from build123d import *

# Parameters (mm, degrees)
SKETCH1_R               = 10
BOSS_EXTRUDE1_DEPTH     = 15
SKETCH2_R               = 12.5
BOSS_EXTRUDE2_DEPTH     = 20
SKETCH3_R               = 12
BOSS_EXTRUDE3_DEPTH     = 139.5
SKETCH4_R               = 4.5
CUT_EXTRUDE1_DEPTH      = 176.393129854
CUT_EXTRUDE2_DEPTH      = 176.393129954
CUT_EXTRUDE2_DEPTH_BACK = 176.393129954
SKETCH5_W               = 50.129657838
SKETCH5_H               = 19.874218845
LPATTERN1_COUNT         = 2
LPATTERN1_PITCH         = 25


with BuildPart() as part:
    # Sketch1 → Boss-Extrude1 (new body)
    with BuildSketch(Plane.XY):
        Circle(SKETCH1_R)
    extrude(amount=BOSS_EXTRUDE1_DEPTH)

    # Sketch2 → Boss-Extrude2 (add)
    with BuildSketch(Plane.XY.offset(15)):
        Circle(SKETCH2_R)
    extrude(amount=BOSS_EXTRUDE2_DEPTH)

    # Sketch3 → Boss-Extrude3 (add)
    with BuildSketch(Plane.XY.offset(35)):
        Circle(SKETCH3_R)
    extrude(amount=BOSS_EXTRUDE3_DEPTH)

    # Sketch4 → Cut-Extrude1 (cut, symmetric)
    with BuildSketch(Plane(origin=(0, 0, 0), x_dir=(1, 0, 0), z_dir=(0, 1, 0))):
        with Locations(Location((0, -154.5, 0), (0, 0, 270))):
            Circle(SKETCH4_R)
    cut_extrude1 = extrude(amount=CUT_EXTRUDE1_DEPTH, both=True, mode=Mode.SUBTRACT)

    # Sketch5 → Cut-Extrude2 (cut, two sides: drawn at the far end of the back side and taken through both)
    with BuildSketch(Plane(origin=(0, 0, 0), x_dir=(1, 0, 0), z_dir=(0, 1, 0)).offset(-CUT_EXTRUDE2_DEPTH_BACK)):
        with Locations((-12.564828919, -5.062890578)):
            Rectangle(SKETCH5_W, SKETCH5_H)
    extrude(amount=CUT_EXTRUDE2_DEPTH + CUT_EXTRUDE2_DEPTH_BACK, mode=Mode.SUBTRACT)

    # LPattern1: Cut-Extrude1 ×2
    with Locations(*[(0, 0, -i * LPATTERN1_PITCH) for i in range(1, LPATTERN1_COUNT)]):
        add(cut_extrude1, mode=Mode.SUBTRACT)


solid = part.part
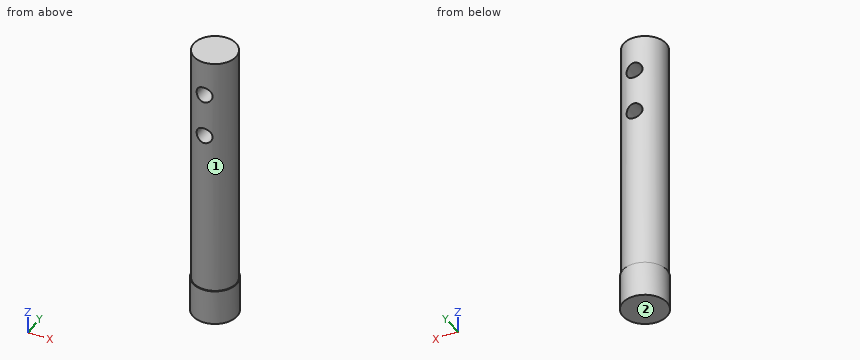
Geometry: final body of the model. Coordinates: model frame, mm. Face numbers are marked on the shaded views. A direction names the side the tool comes from. Coordinates: 2 decimals unless noted, no trailing zeros. Loops run counter-clockwise (first coordinate to the right, second up) from the corner with the lowest first, then second, coordinate; pieces in that order, holes last. Notation, with made-up numbers: (88, 79) - (144, 79) arc R6 ccw to (144, 88) - close; hole circle Ø5 at (-24.75, 2.25). An arc over 180 degrees is marked (long way). Put each result on its own line as item: value. Start each with the question number.
Q1. Line query: line 1 (Z direction, x = 0.5, y = -1.25); line 2 (Z direction, x = -2, y = 5.25); line 3 (X direction, y = -0.5, z = 154.5). Output: solid intervals per line, ascending.
Q2. Set-up query: the marked faces 1 and 2. Return all of +Z, -Z, +X, -X, +Y, -Y with unobstructed straight access to the full face (end or side cutting, diameter ignored); none if empty.
Q3. Pin query (flat end, axial travel): pin 1 Ø14.5 at (x, z) = (0, 129.5) entering from -Y; pin 2 Ø6 at (y, z) = (9, 122) entering from +X; pin 3 Ø5 at (y, z) = (2.5, 105.5) entering from +X. Return the tip coordinate at first contact, or that it passes through.
Q4. Cut plane D-D, the plane y = 6.5. Return loops of the section in (x, z), and give its area (3 significant figures).
Q5. Cut plane C-C, the plane z = 129.5. Return loops of the section in (x, y).
Q6. Cut plane B-B, the plane y = 0. Return loops of the section in (x, z).
Q7. Cut plane A-A, the plane x = 0. Return loops of the section in (y, z).
Filled sheet:
1. line 1: 15 to 125.03, 133.97 to 150.03, 158.97 to 174.5
1. line 2: 15 to 125.47, 133.53 to 150.47, 158.53 to 174.5
1. line 3: -11.99 to -4.5, 4.5 to 11.99
2. face 1: +Z
2. face 2: -Z, +X, -X, +Y, -Y
3. pin 1: y = -12
3. pin 2: x = 10.39
3. pin 3: x = 12
4. outline: (-10.68, 15) - (10.68, 15) - (10.68, 35) - (10.09, 35) - (10.09, 174.5) - (-10.09, 174.5) - (-10.09, 35) - (-10.68, 35) - close; hole circle Ø9 at (0, 129.5); hole circle Ø9 at (0, 154.5)
4. area: 3,110 mm²
5. outline: (-4.5, -11.12) - (-4.5, 11.12) arc R12 ccw to start; (4.5, -11.12) arc R12 ccw to (4.5, 11.12) - close
6. outline: (-12.5, 15) - (12.5, 15) - (12.5, 35) - (12, 35) - (12, 174.5) - (-12, 174.5) - (-12, 35) - (-12.5, 35) - close; hole circle Ø9 at (0, 129.5); hole circle Ø9 at (0, 154.5)
7. outline: (-12.5, 15) - (12.5, 15) - (12.5, 35) - (12, 35) - (12, 125) - (-12, 125) - (-12, 35) - (-12.5, 35) - close; (-12, 134) - (12, 134) - (12, 150) - (-12, 150) - close; (-12, 159) - (12, 159) - (12, 174.5) - (-12, 174.5) - close
